from build123d import *

# Parameters (mm, degrees)
F0_R     = 12.2
F0_R_2   = 4
F1_DEPTH = 7.5
F2_DEPTH = 2


with BuildPart() as f1:
    # F0 (on Top) → F1 (new body)
    with BuildSketch(Plane.XY):
        Circle(F0_R)
        Polygon((7.361216, 0), (3.680608, -6.375), (-3.680608, -6.375), (-7.361216, 0), (-3.680608, 6.375), (3.680608, 6.375), align=None, mode=Mode.SUBTRACT)
        Polygon((-3.680608, -6.375), (3.680608, -6.375), (7.361216, 0), (3.680608, 6.375), (-3.680608, 6.375), (-7.361216, 0), align=None)
        Circle(F0_R_2, mode=Mode.SUBTRACT)
    extrude(amount=F1_DEPTH)

    # F0 (on Top) → F2 (cut)
    with BuildSketch(Plane.XY):
        Circle(F0_R_2)
        Polygon((-3.680608, -6.375), (3.680608, -6.375), (7.361216, 0), (3.680608, 6.375), (-3.680608, 6.375), (-7.361216, 0), align=None)
        Circle(F0_R_2, mode=Mode.SUBTRACT)
    extrude(amount=F2_DEPTH, mode=Mode.SUBTRACT)


solid = f1.part
Design review of the part built by this model. Coordinates are the model's own, in mm. A direction names the side the tool comes from. Coordinates: 2 decimals unless noted, no trailing zeros. Order: outer loops, then holes, each group sorted by start corner. A loop starts at its lowest first (then second) coordinate and runs counter-clockwise, first axis right, second up. Notation, with made-up numbers: (-37.5, 59.25) -> (-16.5, 59.25) arc R15 ccw to (-16.5, 80.25) -> close; hole circle Ø4 at (45, 57). An arc over 180 degrees is marked (long way). Use one line per item in the form item = value. Start each with the question number.
(1) For faces 4 (the flat face through (-3, 3, 7.5)), 5 (the flat face through (0, 6.375, 1)), list the 3-axis set-ups (+Z, -Z, +X, -X, +Y, -Y) from which the entire face can be reached by the end or side of a thin tool; tool diameter is ignored.
(2) Add section C-C on z = 5.5. State the section outline as (x, y) points.
(3) The part is to be moulded in two halves that separate along X. For faces 1 (the cylindrical face through (-12.19, 0.54, 3.7)), 2 (the flat face through (-5.495, 3.232, 0.986)), 3 (the flat face through (5, -5, 0)), say which applies: +X half, -X half, draft (parallel to the pull), parting line (faces both ways), or undercut.
(4) Insertion check: pin 1 (1.6 mm diameter, centred on x = -2, z = 0.5, fed in from +Y); pin 2 (1.6 mm diameter, centred on x = -1.5, z = 1.5, fed in from -Y); pin 3 (10.5 mm diameter, centred on x = 0, y = 0, fed in from +Z); pin 4 (1.5 mm diameter, centred on y = -3.5, z = 3.5, fed in from +X). Each pin has a flat end and moves straight along its axis. Give the tip position at first contact, or say it passes through.
(5) Add section B-B on y = -0.75. State the section outline as (x, z) points, plus the area to 3 significant figures.
(6) Add section D-D on y = -4.75. State the section outline as (x, z) points.
(7) Add section A-A on x = 0. State the section outline as (y, z) points (3 decimals).
(8) For probe 1 along Y at (x, z) = (0, 4.1); probe 2 along Z at (x, y) = (4, -5.75); probe 3 along Y at (x, z) = (3.5, 0.75) (3 decimals), list the stretches that pass through material, from the lowest coordinate up.
Answer block:
q1.face_4 = +Z, +X, -X, +Y, -Y
q1.face_5 = -Z
q2.outline = circle Ø24.4 at (0, 0); hole circle Ø8 at (0, 0)
q3.face_1 = parting line
q3.face_2 = undercut
q3.face_3 = draft
q4.pin_1 = 12.14
q4.pin_2 = -12.18
q4.pin_3 = 7.5
q4.pin_4 = 11.89
q5.outline = (-12.18, 0) -> (-6.93, 0) -> (-6.93, 2) -> (-3.93, 2) -> (-3.93, 7.5) -> (-12.18, 7.5) -> close; (3.93, 2) -> (6.93, 2) -> (6.93, 0) -> (12.18, 0) -> (12.18, 7.5) -> (3.93, 7.5) -> close
q5.area = 112 mm²
q6.outline = (-11.24, 0) -> (-4.62, 0) -> (-4.62, 2) -> (4.62, 2) -> (4.62, 0) -> (11.24, 0) -> (11.24, 7.5) -> (-11.24, 7.5) -> close
q7.outline = (-12.2, 0) -> (-6.375, 0) -> (-6.375, 2) -> (-4, 2) -> (-4, 7.5) -> (-12.2, 7.5) -> close; (4, 2) -> (6.375, 2) -> (6.375, 0) -> (12.2, 0) -> (12.2, 7.5) -> (4, 7.5) -> close
q8.probe_1 = -12.2 to -4, 4 to 12.2
q8.probe_2 = 2 to 7.5
q8.probe_3 = -11.687 to -6.375, 6.375 to 11.687
